```python
from build123d import *

# Parameters (mm, degrees)
EXTRUDE_1_DEPTH     = 12
SKETCH_2_R          = 2.55
CUT_EXTRUDE_1_DEPTH = 19
CUT_EXTRUDE_2_DEPTH = 19
SKETCH_4_R          = 1
CUT_EXTRUDE_3_DEPTH = 19
SKETCH_5_W          = 10
SKETCH_5_H          = 2
CUT_EXTRUDE_4_DEPTH = 19
SKETCH_6_R          = 7
CUT_EXTRUDE_5_DEPTH = 19
CUT_EXTRUDE_6_DEPTH = 19


with BuildPart() as part:
    # 草图1 → 凸台-拉伸1 (new body)
    with BuildSketch(Plane.XY):
        Polygon((0, 0), (35, 0), (35, -3.5), (47, -3.5), (47, -6.5), (35, -6.5), (35, -9.5), (47, -9.5), (47, -12.5), (35, -12.5), (35, -15.5), (47, -15.5), (47, -18.5), (35, -18.5), (35, -22), (0, -22), (0, -17), (-10, -17), (-10, -12), (0, -12), (0, -10), (-10, -10), (-10, -5), (0, -5), align=None)
    extrude(amount=EXTRUDE_1_DEPTH)

    # 草图2 → 切除-拉伸1 (cut)
    with BuildSketch(Plane(origin=(0, -3.5, 0), x_dir=(1, 0, 0), z_dir=(0, 1, 0))):
        with Locations((42, -6)):
            Circle(SKETCH_2_R)
    extrude(amount=-CUT_EXTRUDE_1_DEPTH, mode=Mode.SUBTRACT)

    # 草图3 → 切除-拉伸2 (cut)
    with BuildSketch(Plane(origin=(0, -3.5, 0), x_dir=(1, 0, 0), z_dir=(0, 1, 0))):
        with BuildLine():
            Line((42, -1), (35, -1))
            Line((35, -1), (35, 1.362905895))
            Line((35, 1.362905895), (53.328864927, 1.362905895))
            Line((53.328864927, 1.362905895), (53.328864927, -14.813237877))
            Line((53.328864927, -14.813237877), (35, -14.813237877))
            Line((35, -14.813237877), (35, -11))
            Line((35, -11), (42, -11))
            ThreePointArc((42, -11), (47, -6), (42, -1))
        make_face()
    extrude(amount=-CUT_EXTRUDE_2_DEPTH, mode=Mode.SUBTRACT)

    # 草图4 → 切除-拉伸3 (cut)
    with BuildSketch(Plane.XZ.offset(17)):
        with Locations((-2.5, 6)):
            Circle(SKETCH_4_R)
    extrude(amount=-CUT_EXTRUDE_3_DEPTH, mode=Mode.SUBTRACT)

    # 草图5 → 切除-拉伸4 (cut)
    with BuildSketch(Plane.XY.offset(12)):
        with Locations((5, -11)):
            Rectangle(SKETCH_5_W, SKETCH_5_H)
    extrude(amount=-CUT_EXTRUDE_4_DEPTH, mode=Mode.SUBTRACT)

    # 草图6 → 切除-拉伸5 (cut)
    with BuildSketch(Plane.XY.offset(12)):
        with Locations((10, -11)):
            Circle(SKETCH_6_R)
    extrude(amount=-CUT_EXTRUDE_5_DEPTH, mode=Mode.SUBTRACT)

    # 草图7 → 切除-拉伸6 (cut)
    with BuildSketch(Plane(origin=(0, -5, 0), x_dir=(1, 0, 0), z_dir=(0, 1, 0))):
        with BuildLine():
            Line((-3, -12), (-3, -16.245470045))
            Line((-3, -16.245470045), (-15.241663488, -16.245470045))
            Line((-15.241663488, -16.245470045), (-15.241663488, 3.326156632))
            Line((-15.241663488, 3.326156632), (-3, 3.326156632))
            Line((-3, 3.326156632), (-3, 0))
            ThreePointArc((-3, 0), (-5.395390723, -6), (-3, -12))
        make_face()
    extrude(amount=-CUT_EXTRUDE_6_DEPTH, mode=Mode.SUBTRACT)


solid = part.part
```
Work out the finished part from the listing and answer in its coordinate system (mm). A direction names the side the tool comes from. Coordinates: 2 decimals unless noted, no trailing zeros. Write each loop counter-clockwise with the first axis right and the second up, starting at its lowest first coordinate (ties: lowest second). Pieces come first, ordered by that corner, then holes.
Q1. A cutting plane is placed at D-D, the plane z = 6. State how many separate pieces and enclosed holes the cut face has, then the cut area to 3 significant figures.
Q2. A cutting plane is placed at A-A, the plane x = 37.5. Give the vertices of the cut face in (y, z), then the cut area to 3 significant figures.
Q3. Which of the six approach directions +Z, -Z, +X, -X, +Y, -Y give full straight-line access (tool end or side, diameter ignored) to faces 1 (the face through (-1, -17, 6)), 2 (the face through (39, -5, 1)), 3 (the face through (38, -15.5, 6)), 4 (the face through (-2.1, -5, 4.6))?
Q4. A cutting plane is placed at B-B, the plane y = -16. Give the vertices of the cut face in (x, z), then the cut area to 3 significant figures.
Q5. Each of these flat-tipped pins is pushed along its axis until it touches: pin 1 Ø5 at (x, z) = (40.5, 5) entering from +Y; pin 2 Ø1.5 at (x, y) = (40, -16.5) entering from -Z; pin 3 Ø5 at (x, z) = (40.5, 7.5) entering from -Y. Where does it stop, or does it pass through?
Q6. A cutting plane is placed at C-C, the plane x = -2.5. Give the vertices of the cut face in (y, z), then the cut area to 3 significant figures.
Q7. Find the intervals of material crossed by line 1 (Y direction, x = 44, z = 9.5); line 2 (Y direction, x = -2, z = 10); line 3 (X direction, y = -10.95, z = 6), in increasing order.
Q8. Determine the mould class of faces 5 (the face through (17, 0, 6)), 6 (the face through (47, -11, 6)), 7 (the face through (39.452, -16.979, 5.888)), 8 (the face through (0, -3, 6)) for opening direction X: released by +X, released by -X, zero draft, split by the parting line, or undercut.
Findings below:
1. separate pieces: 6
1. enclosed holes: 0
1. area: 706 mm2
2. outline: (-18.5, 1) - (-15.5, 1) - (-15.5, 11) - (-18.5, 11) - close; (-12.5, 1) - (-9.5, 1) - (-9.5, 11) - (-12.5, 11) - close; (-6.5, 1) - (-3.5, 1) - (-3.5, 11) - (-6.5, 11) - close
2. area: 90.0 mm2
3. face 1: +Z, -Z, -X, -Y
3. face 2: -Z, +X, +Y, -Y
3. face 3: +Z, -Z, +X
3. face 4: +Z, -Z, -X, +Y
4. outline: (-3, 0) - (5.1, 0) - (5.1, 12) - (-3, 12) arc R8.71 ccw to start; (14.9, 0) - (35, 0) - (35, 1) - (42, 1) arc R5 ccw to (42, 11) - (35, 11) - (35, 12) - (14.9, 12) - close; hole circle Ø2 at (-2.5, 6); hole circle Ø5.1 at (42, 6)
4. area: 444 mm2
5. pin 1: stops at y = -3.5
5. pin 2: stops at z = 1
5. pin 3: stops at y = -18.5
6. outline: (-17, 0) - (-12, 0) - (-12, 5) - (-17, 5) - close; (-17, 7) - (-12, 7) - (-12, 12) - (-17, 12) - close; (-10, 0) - (-5, 0) - (-5, 5) - (-10, 5) - close; (-10, 7) - (-5, 7) - (-5, 12) - (-10, 12) - close
6. area: 100 mm2
7. line 1: y = -18.5 to -15.5, -12.5 to -9.5, -6.5 to -3.5
7. line 2: y = -17 to -12, -10 to -5
7. line 3: x = 17 to 39.45, 44.55 to 47
8. face 5: zero draft
8. face 6: released by +X
8. face 7: undercut
8. face 8: released by -X
